Can you work these out from the model? Positions are in its coordinate system, mm. A direction names the side the tool comes from. Round coordinates to 2 decimals unless told otherwise and drop trailing zeros. Loops run counter-clockwise (first coordinate to the right, second up) from the corner with the lowest first, then second, coordinate; pieces in that order, holes last. Notation, with made-up numbers: (-20.5, 46) -> (35.5, 46) arc R29 ccw to (35.5, 85) -> close; hole circle Ø8 at (54.25, 37). An arc over 180 degrees is marked (long way). Write item = value, one per line.
from build123d import *

# Parameters (mm, degrees)
F_1_16_NPT_TAPPED_HOLE1_AT_2_COUNT = 2
F_1_16_NPT_TAPPED_HOLE1_AT_2_PITCH = 24.248711306
F_1_16_NPT_TAPPED_HOLE1_AT_3_COUNT = 2
F_1_16_NPT_TAPPED_HOLE1_AT_3_PITCH = 24.248711306
THRUST_MOUNT_DEPTH                 = 6
SKETCH6_R                          = 1
LOCKING_PIN_DEPTH                  = 48.340521755
CIRPATTERN1_COUNT                  = 3
SKETCH7_W                          = 0.5
SKETCH7_H                          = 1
F_2_2_2_2_DIAMETER_HOLE1_D         = 2.2
CIRPATTERN2_COUNT                  = 6


with BuildPart() as part:
    # Sketch1 → Main Base (revolve)
    with BuildSketch(Plane(origin=(0, 0, 0), x_dir=(0, 0, -1), z_dir=(1, 0, 0))):
        with BuildLine():
            Line((0, 31.75), (0, 24.479181))
            ThreePointArc((0, 24.479181), (-2.722361108, 23.351542108), (-3.85, 20.629181))
            Line((-3.85, 20.629181), (-3.85, 8))
            Line((-3.85, 8), (-5.004700538, 6))
            Line((-5.004700538, 6), (-15, 6))
            Line((-15, 6), (-15, 8))
            Line((-15, 8), (-11.85, 8))
            Line((-11.85, 8), (-11.85, 20.629181))
            Line((-11.85, 20.629181), (-5.85, 20.629181))
            ThreePointArc((-5.85, 20.629181), (-4.791789853, 23.984959598), (-2, 26.126680432))
            Line((-2, 26.126680432), (-2, 31.75))
            Line((-2, 31.75), (0, 31.75))
        make_face()
    revolve(axis=Axis((0, 0, -128.05411072), (0, 0, 1)))

    # Sketch4 → 1/16 NPT Tapped Hole1 (revolve, cut)
    with BuildSketch(Plane(origin=(0, 14, 11.85), x_dir=(0, -1, 0), z_dir=(1, 0, 0))):
        Polygon((0, 0), (0, 8), (3.0734, 8), (3.0734, 6.89), (3.364817173, 6.89), (3.571113, 0), align=None)
    f_1_16_npt_tapped_hole1 = revolve(axis=Axis((0, 14, 18.2), (0, 0, -1)), mode=Mode.SUBTRACT)

    # 1/16 NPT Tapped Hole1 at 2: 1/16 NPT Tapped Hole1 ×2
    with Locations(*[Vector(0.5000000000000264, -0.8660254037844235, 0) * (i * F_1_16_NPT_TAPPED_HOLE1_AT_2_PITCH) for i in range(1, F_1_16_NPT_TAPPED_HOLE1_AT_2_COUNT)]):
        add(f_1_16_npt_tapped_hole1, mode=Mode.SUBTRACT)

    # 1/16 NPT Tapped Hole1 at 3: 1/16 NPT Tapped Hole1 ×2
    with Locations(*[Vector(-0.4999999999999739, -0.8660254037844536, 0) * (i * F_1_16_NPT_TAPPED_HOLE1_AT_3_PITCH) for i in range(1, F_1_16_NPT_TAPPED_HOLE1_AT_3_COUNT)]):
        add(f_1_16_npt_tapped_hole1, mode=Mode.SUBTRACT)

    # Sketch5 → Thrust Mount (cut)
    with BuildSketch(Plane.XY.offset(11.85)):
        with BuildLine():
            Line((25.617872251, 10.207767679), (14.081667359, 3.547336679))
            ThreePointArc((14.081667359, 3.547336679), (8.660254038, 5), (10.112917359, 10.421413321))
            Line((10.112917359, 10.421413321), (21.649122251, 17.081844321))
            ThreePointArc((21.649122251, 17.081844321), (27.070535573, 15.629181), (25.617872251, 10.207767679))
        make_face()
        with BuildLine():
            Line((-3.96875, -28.289612), (-3.96875, -12.96875))
            ThreePointArc((-3.96875, -12.96875), (0, -9), (3.96875, -12.96875))
            Line((3.96875, -12.96875), (3.96875, -28.289612))
            ThreePointArc((3.96875, -28.289612), (0, -32.258362), (-3.96875, -28.289612))
        make_face()
        with BuildLine():
            Line((-21.649122251, 17.081844321), (-10.112917359, 10.421413321))
            ThreePointArc((-10.112917359, 10.421413321), (-8.660254038, 5), (-14.081667359, 3.547336679))
            Line((-14.081667359, 3.547336679), (-25.617872251, 10.207767679))
            ThreePointArc((-25.617872251, 10.207767679), (-27.070535573, 15.629181), (-21.649122251, 17.081844321))
        make_face()
    extrude(amount=-THRUST_MOUNT_DEPTH, mode=Mode.SUBTRACT)

    # Sketch6 → Locking Pin (cut, symmetric)
    with BuildSketch(Plane(origin=(0, 0, 0), x_dir=(0, 0, -1), z_dir=(1, 0, 0))):
        with Locations((-8.85, -16.243817134)):
            Circle(SKETCH6_R)
    locking_pin = extrude(amount=LOCKING_PIN_DEPTH, both=True, mode=Mode.SUBTRACT)

    # CirPattern1: Locking Pin ×3 about axis
    cirpattern1_axis = Axis((0, 0, 55), (0, 0, -1))
    for i in range(1, CIRPATTERN1_COUNT):
        add(locking_pin.rotate(cirpattern1_axis, i * 360 / CIRPATTERN1_COUNT), mode=Mode.SUBTRACT)

    # Sketch7 → Face O-ring (revolve, cut)
    with BuildSketch(Plane(origin=(0, 0, 0), x_dir=(0, 0, -1), z_dir=(1, 0, 0)), mode=Mode.PRIVATE) as face_o_ring_sk:
        with Locations((-0.25, 26.479181)):
            Rectangle(SKETCH7_W, SKETCH7_H)
    revolve(face_o_ring_sk.sketch.rotate(Axis((0, 0, 55), (0, 0, -1)), 90), axis=Axis((0, 0, 55), (0, 0, -1)), mode=Mode.SUBTRACT)

    # Ø2.2 (2.2) Diameter Hole1 (through all)
    with Locations(Plane.XY.offset(2)):
        with Locations((0, 29)):
            f_2_2_2_2_diameter_hole1 = Hole(F_2_2_2_2_DIAMETER_HOLE1_D / 2)

    # CirPattern2: Ø2.2 (2.2) Diameter Hole1 ×6 about axis
    cirpattern2_axis = Axis((0, 0, 0), (0, 0, 1))
    for i in range(1, CIRPATTERN2_COUNT):
        add(f_2_2_2_2_diameter_hole1.rotate(cirpattern2_axis, i * 360 / CIRPATTERN2_COUNT), mode=Mode.SUBTRACT)


solid = part.part
1. For faces 4 (the flat face through (3.969, -17.4, 8.9)), 5 (the cylindrical face through (-17.987, -10.1, 8.808)), 6 (the cylindrical face through (-19.148, -17.558, 0.246)), 7 (the flat face through (-12, 24, 2)), which set-ups out of +Z, -Z, +X, -X, +Y, -Y let a thin tool reach every point of the face, with its end or its side?
Entries:
face_4 = +Z, -Y
face_5 = +Z, -X
face_6 = -Z
face_7 = +Z
2. I need wall thicknesses on line 1 (Y direction, x = -11, z = 7.5); line 2 (X direction, y = -4, z = 10.5); line 3 (Z direction, x = -17.5, y = 9.5). Which ranges of each line are inside material? Lowest first, please. Write a range as [from, to].
Entries:
line_1 = [-17.45, -10.25], [-3.75, 3.17], [10.93, 17.45]
line_2 = [-20.24, -13.99], [-10.26, -4.47], [4.47, 10.26], [13.99, 20.24]
line_3 = [3.85, 5.85]
3. I'm going to push flat-ended pins straight in: pin 1 (1.6 mm diameter, centred on y = -16.24, z = 8.85, fed in from +X); pin 2 (6.5 mm diameter, centred on x = -0.5, y = -14.5, fed in from +Z); pin 3 (1.5 mm diameter, centred on x = -3.5, z = 11, fed in from +Y); pin 4 (8 mm diameter, centred on x = 0, y = 14, fed in from -Z). Where does each tip first touch, or does it pass through?
Entries:
pin_1 = through
pin_2 = 5.85
pin_3 = 20.45
pin_4 = 3.85
4. Suppose I cut it at D-D, the plane z = 14.25. List the corners of the cut face in (x, y) for me.
Entries:
outline = circle Ø16 at (0, 0); hole circle Ø12 at (0, 0)
5. Suppose I cut it at A-A, the plane z = 8.85. Count the separate pieces of the cut face and the enclosed holes in it, and give its area (3 significant figures).
Entries:
separate_pieces = 7
enclosed_holes = 4
area = 767 mm²
6. We'd pull the mould along Y, two halves only. Please class faces 1 (the cylindrical face through (0.247, 20.628, 8.808)), 2 (the cylindrical face through (17.74, -10.53, 8.81)), 3 (the flat face through (13.4, 12.32, 8.89)): released by +Y, released by -Y, zero draft, split by the parting line, or undercut.
Entries:
face_1 = released by +Y
face_2 = split by the parting line
face_3 = undercut
